Could you check a few things on this model? Use its own coordinates, in mm. Give positions to 0.01 mm unless a question says otherwise; leave off trailing zeros. Loops run counter-clockwise (first coordinate to the right, second up) from the corner with the lowest first, then second, coordinate; pieces in that order, holes last. Notation, with made-up numbers: M 76.25,53 L 93.25,53 A23 ccw 93.25,66 Z; hole C 87,1 d7. An arc over 180 degrees is marked long. Return JSON: item names as keys, results as strings. Group by question number.
1. Please list where these lines run through material, in increasing order: line 1 (Z direction, x = 2, y = -5.5); line 2 (Z direction, x = -12, y = -2.5); line 3 (X direction, y = -5, z = 73).
2. If we section it at B-B (z = -97): Write out the boundary of the cut face in (x, y), plus the area to 3 significant figures.
3. If we section it at C-C (x = 123.5): Write out the boundary of the cut face in (y, z), plus the area to 3 significant figures.
4. For pin 1 (2 mm diameter, centred on y = -4.5, z = -3.5, fed in from -X); pin 2 (3 mm diameter, centred on y = -3, z = -96, fed in from +X); pin 3 (3 mm diameter, centred on y = -1, z = 26, fed in from +X), each with a flat end and sliding along its axis, tell me the tip position at first contact or that it passes through.
5. If we mould it in two halves opening along Z, with no side actions, what happens to faces 1 (the cylindrical face through (-153.267, -3.131, -34.035)), 2 (the cylindrical face through (7.509, -3.131, 23.846)), 3 (the flat face through (-33, -6.35, -2))? For each: +Z half, -Z half, draft (parallel to the pull), parting line (faces both ways), or undercut.
6. If we section it at A-A (y = -1): State how many separate pieces and enclosed holes the cut face has, plus the area to 3 significant figures.
```python
from build123d import *

# Parameters (mm, degrees)
SKETCH2_R           = 157
BOSS_EXTRUDE1_DEPTH = 6.35
SKETCH4_R           = 25
CUT_EXTRUDE1_DEPTH  = 223.122314278
SKETCH5_R           = 1.7
CUT_EXTRUDE2_DEPTH  = 223.122314278
CIRPATTERN1_COUNT   = 4
SKETCH7_R           = 1.7
CUT_EXTRUDE4_DEPTH  = 223.122314278
CIRPATTERN2_COUNT   = 11
CIRPATTERN2_ANGLE   = 150


with BuildPart() as part:
    # Sketch2 → Boss-Extrude1 (new body)
    with BuildSketch(Plane(origin=(0, 0, 0), x_dir=(1, 0, 0), z_dir=(0, 1, 0))):
        with Locations(Location((0, 0, 0), (0, 0, 270))):
            Circle(SKETCH2_R)
    extrude(amount=-BOSS_EXTRUDE1_DEPTH)

    # Sketch4 → Cut-Extrude1 (cut, through all)
    with BuildSketch(Plane(origin=(0, 0, 0), x_dir=(1, 0, 0), z_dir=(0, 1, 0))):
        with Locations(Location((0, 0, 0), (0, 0, 270))):
            Circle(SKETCH4_R)
    extrude(amount=-CUT_EXTRUDE1_DEPTH, mode=Mode.SUBTRACT)

    # Sketch5 → Cut-Extrude2 (cut, through all)
    with BuildSketch(Plane.XZ.offset(6.35)):
        with Locations(Location((0, 45, 0), (0, 0, 270))):
            Circle(SKETCH5_R)
    cut_extrude2 = extrude(amount=-CUT_EXTRUDE2_DEPTH, mode=Mode.SUBTRACT)

    # CirPattern1: Cut-Extrude2 ×4 about axis
    cirpattern1_axis = Axis((0, 0, 0), (0, 1, 0))
    for i in range(1, CIRPATTERN1_COUNT):
        add(cut_extrude2.rotate(cirpattern1_axis, i * 360 / CIRPATTERN1_COUNT), mode=Mode.SUBTRACT)

    # Sketch7 → Cut-Extrude4 (cut, through all)
    with BuildSketch(Plane(origin=(0, 0, 0), x_dir=(1, 0, 0), z_dir=(0, 1, 0))):
        with Locations(Location((-146.820725596, 39.340494856, 0), (0, 0, 270))):
            Circle(SKETCH7_R)
    cut_extrude4 = extrude(amount=-CUT_EXTRUDE4_DEPTH, mode=Mode.SUBTRACT)

    # CirPattern2: Cut-Extrude4 ×11 about axis
    cirpattern2_axis = Axis((0, 0, 0), (0, -1, 0))
    for i in range(1, CIRPATTERN2_COUNT):
        add(cut_extrude4.rotate(cirpattern2_axis, i * CIRPATTERN2_ANGLE / (CIRPATTERN2_COUNT - 1)), mode=Mode.SUBTRACT)


solid = part.part
```
Answer:
{
 "1": {"line 1": "z = -156.99 to -24.92, 24.92 to 156.99", "line 2": "z = -156.54 to -21.93, 21.93 to 156.54", "line 3": "x = -139 to 139"},
 "2": {"outline": "M -123.45,-6.35 L 123.45,-6.35 L 123.45,0 L -123.45,0 Z", "area": "1,570 mm²"},
 "3": {"outline": "M -6.35,-96.94 L 0,-96.94 L 0,96.94 L -6.35,96.94 Z", "area": "1,230 mm²"},
 "4": {"pin 1": "stops at x = -156.98", "pin 2": "stops at x = 125.37", "pin 3": "stops at x = 155.08"},
 "5": {"face 1": "parting line", "face 2": "undercut", "face 3": "draft"},
 "6": {"separate pieces": "1", "enclosed holes": "16", "area": "75,300 mm²"}
}
